from build123d import *

# Parameters (mm, degrees)
SKETCH1_R           = 9.5
SKETCH1_R_2         = 4
SKETCH1_R_3         = 1
BOSS_EXTRUDE1_DEPTH = 2.5
BOSS_EXTRUDE2_DEPTH = 2.5
CIRPATTERN1_COUNT   = 15


with BuildPart() as part:
    # Sketch1 → Boss-Extrude1 (new body)
    with BuildSketch(Plane.XY):
        Circle(SKETCH1_R)
        Circle(SKETCH1_R_2, mode=Mode.SUBTRACT)
        with Locations((0, 7)):
            Circle(SKETCH1_R_3, mode=Mode.SUBTRACT)
        with Locations((7, 0)):
            Circle(SKETCH1_R_3, mode=Mode.SUBTRACT)
        with Locations((0, -7)):
            Circle(SKETCH1_R_3, mode=Mode.SUBTRACT)
        with Locations((-7, 0)):
            Circle(SKETCH1_R_3, mode=Mode.SUBTRACT)
    extrude(amount=BOSS_EXTRUDE1_DEPTH)

    # Sketch2 → Boss-Extrude2 (add)
    with BuildSketch(Plane.XY):
        Polygon((-1.5, 9.38083152), (-0.633974596, 10.88083152), (0.633974596, 10.88083152), (1.5, 9.38083152), align=None)
    boss_extrude2 = extrude(amount=BOSS_EXTRUDE2_DEPTH)

    # CirPattern1: Boss-Extrude2 ×15 about axis
    cirpattern1_axis = Axis((0, 0, 0), (0, 0, 1))
    for i in range(1, CIRPATTERN1_COUNT):
        add(boss_extrude2.rotate(cirpattern1_axis, i * 360 / CIRPATTERN1_COUNT))


solid = part.part
Verification items for the finished model (mm, model axes). A direction names the side the tool comes from. Coordinates: 2 decimals unless noted, no trailing zeros. Order: outer loops, then holes, each group sorted by start corner. A loop starts at its lowest first (then second) coordinate and runs counter-clockwise, first axis right, second up.
Item 1: Section check D-D, the plane y = -4.5. Enter the section's corners in (x, z), then the cut area to 3 significant figures.
Filled in:
outline: (-9.51, 0) - (9.51, 0) - (9.51, 2.5) - (-9.51, 2.5) - close
area: 47.6 mm2
Item 2: Section check A-A, the plane x = 0. Enter the section's corners in (y, z), then the cut area to 3 significant figures.
Filled in:
outline: (-9.5, 0) - (-8, 0) - (-8, 2.5) - (-9.5, 2.5) - close; (-6, 0) - (-4, 0) - (-4, 2.5) - (-6, 2.5) - close; (4, 0) - (6, 0) - (6, 2.5) - (4, 2.5) - close; (8, 0) - (10.88, 0) - (10.88, 2.5) - (8, 2.5) - close
area: 21.0 mm2
Item 3: Section check B-B, the plane y = -7. Enter the section's corners in (x, z), then the cut area to 3 significant figures.
Filled in:
outline: (-6.76, 0) - (-1, 0) - (-1, 2.5) - (-6.76, 2.5) - close; (1, 0) - (6.76, 0) - (6.76, 2.5) - (1, 2.5) - close
area: 28.8 mm2
Item 4: Depth check by flat-ended pin: pin 1 (0.5 mm diameter, centred on x = 8, z = 2, fed in from -Y); pin 2 (1.8 mm diameter, centred on x = 0, y = 7, fed in from -Z). Enter the tip coordinate at first touch or a pass-through.
Filled in:
pin 1: stops at y = -5.99
pin 2: passes through
Item 5: Section check C-C, the plane z = 1.3. Give the number of separate pieces and of enclosed holes in the cut face, then the cut area to 3 significant figures.
Filled in:
separate pieces: 1
enclosed holes: 5
area: 265 mm2
Item 6: Material ranges on L1, parallel to Y at x = 0, z = 1.2; L2, parallel to X at y = 6.5, z = 1.85; L3, parallel to X at y = -3, z = 2.15, recorded low to high.
Filled in:
L1: y = -9.5 to -8, -6 to -4, 4 to 6, 8 to 10.88
L2: x = -8.41 to -0.87, 0.87 to 8.41
L3: x = -9.01 to -2.65, 2.65 to 9.01
Item 7: Access from +Z, -Z, +X, -X, +Y, -Y to the whole of each face (thin tool, end or side, straight path). Record for faces 1 (the face through (-9.953, -2.125, 1.232)), 2 (the face through (-8, -5.989, 1)), 3 (the face through (1.98, 9.29, 1.23)), 4 (the face through (8.246, 5.997, 1.232)).
Filled in:
face 1: +Z, -Z, -X
face 2: +Z, -Z, -X, -Y
face 3: +Z, -Z, +Y
face 4: +Z, -Z, +X
Item 8: Release check for a two-part mould opening along X. For faces 5 (the face through (-10.197, -0.005, 1.232)), 6 (the face through (5.103, -8.828, 1.232)), 7 (the face through (0, 10.881, 1)), 8 (the face through (2.27, -10.64, 1.23)) record: +X half, -X half, draft (parallel to the pull), parting line (faces both ways), or undercut.
Filled in:
face 5: -X half
face 6: undercut
face 7: draft
face 8: +X half
